For this review, use the dimensioned drawing (mm, ordinates from the lowest corner) and the shaded views. Give positions to 0.01 mm unless a question says otherwise; leave off trailing zeros. Loops run counter-clockwise (first coordinate to the right, second up) from the corner with the lowest first, then second, coordinate; pieces in that order, holes last. Notation, with made-up numbers: (28.25, 73) -> (60.25, 73) arc R9 ccw to (60.25, 82) -> close; hole circle Ø3 at (-21.75, 14). An arc over 180 degrees is marked (long way). Use a Markdown table: item, result. Add a question column.
1. Add section D-D (x = 7.5). State the section outline as (y, z) points.
2. Draft analysis for pull direction Y (two halves, no side actions). For the marked faces 1, 2 and 3, state which applies: pulls with the +Y half, pulls with the -Y half, needs draft (parallel to the pull), parting line crosses it, or undercut.
3. For pin 1 Ø1.5 at (y, z) = (8.5, 1) entering from +X; pin 2 Ø1 at (x, y) = (19, 3) entering from +Z; pin 3 Ø1 at (x, y) = (14.5, 6) entering from +Z, all flat-tipped, find the tip position at first contact; note any pin that passes through.
4. To check wall thickness, follow line 1 (Y direction, x = 12.7, z = 1.3); line 2 (Y direction, x = 12.75, z = 2.6) (1 decimal); line 3 (X direction, y = 5.75, z = 1.3). State the ranges of each line that lie inside material, in increasing order.
5. Add section A-A (x = 12.7). State the section outline as (y, z) points (1 decimal).
6. Add section C-C (y = 4.75). State the section outline as (x, z) points (1 decimal).
7. Add section B-B (z = 2.1). State the section outline as (x, y) points (1 decimal), and give its area (3 significant figures).
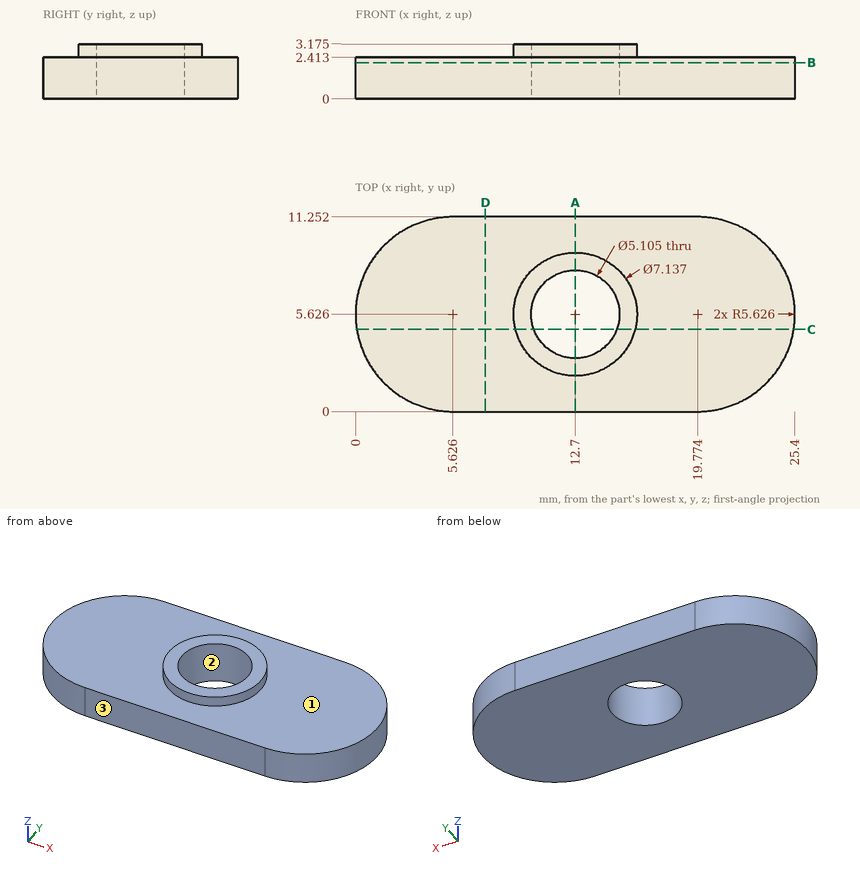
Taken from the geometry:
| question | item | result |
|---|---|---|
| 1 | outline | (0, 0) -> (11.25, 0) -> (11.25, 2.41) -> (0, 2.41) -> close |
| 2 | face 1 | needs draft |
| 2 | face 2 | undercut |
| 2 | face 3 | pulls with the -Y half |
| 3 | pin 1 | stops at x = 24.98 |
| 3 | pin 2 | stops at z = 2.41 |
| 3 | pin 3 | passes through |
| 4 | line 1 | y = 0 to 3.07, 8.18 to 11.25 |
| 4 | line 2 | y = 2.1 to 3.1, 8.2 to 9.2 |
| 4 | line 3 | x = 0 to 10.15, 15.25 to 25.4 |
| 5 | outline | (0, 0) -> (3.1, 0) -> (3.1, 3.2) -> (2.1, 3.2) -> (2.1, 2.4) -> (0, 2.4) -> close; (8.2, 0) -> (11.3, 0) -> (11.3, 2.4) -> (9.2, 2.4) -> (9.2, 3.2) -> (8.2, 3.2) -> close |
| 6 | outline | (0.1, 0) -> (10.3, 0) -> (10.3, 3.2) -> (9.2, 3.2) -> (9.2, 2.4) -> (0.1, 2.4) -> close; (15.1, 0) -> (25.3, 0) -> (25.3, 2.4) -> (16.2, 2.4) -> (16.2, 3.2) -> (15.1, 3.2) -> close |
| 7 | outline | (5.6, 0) -> (19.8, 0) arc R5.6 ccw to (19.8, 11.3) -> (5.6, 11.3) arc R5.6 ccw to start; hole circle Ø5.1 at (12.7, 5.6) |
| 7 | area | 238 mm^2 |
